from build123d import *

# Parameters (mm, degrees)
SKETCH1_R           = 2.5
BOSS_EXTRUDE1_DEPTH = 2


with BuildPart() as part:
    # Sketch1 → Boss-Extrude1 (new body)
    with BuildSketch(Plane(origin=(0, 0, 0), x_dir=(1, 0, 0), z_dir=(0, 1, 0))):
        with BuildLine():
            Line((0, 6), (110, 6))
            ThreePointArc((110, 6), (116, 0), (110, -6))
            Line((110, -6), (0, -6))
            ThreePointArc((0, -6), (-6, 0), (0, 6))
        make_face()
        with Locations(Location((0, 0, 0), (0, 0, 270))):
            Circle(SKETCH1_R, mode=Mode.SUBTRACT)
        with BuildLine():
            Line((10, 2), (110, 2))
            ThreePointArc((110, 2), (112, 0), (110, -2))
            Line((110, -2), (10, -2))
            ThreePointArc((10, -2), (8, 0), (10, 2))
        make_face(mode=Mode.SUBTRACT)
    extrude(amount=BOSS_EXTRUDE1_DEPTH)


solid = part.part
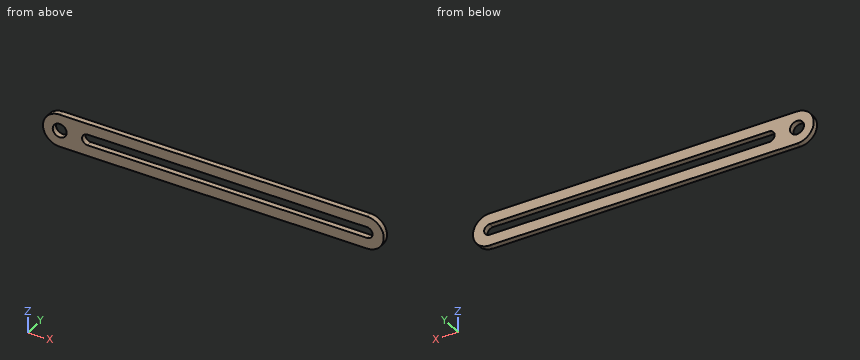
Input: part model. Units: mm. Frame: model coordinates. Coordinates: 2 decimals unless noted, no trailing zeros. Write each loop counter-clockwise with the first axis right and the second up, starting at its lowest first coordinate (ties: lowest second). Pieces come first, ordered by that corner, then holes. Notation, with made-up numbers: M 16.5,-0.75 L 38.5,-0.75 A27 cw 38.5,24.25 Z; hole C 39,-38.5 d2. An arc over 180 degrees is marked long. Answer as a JSON object with one key per item and string values. Group by question number.
(1) Section D-D on z = 4.5. Output: boundary loops of the cut face in (x, y), plus the area to 3 significant figures.
(2) Contact query for a flat-ended pin moving along its axis: P1, Ø1.5, axis at x = 19, z = 2, coming from the -Y side. Output: stop coordinate, or through.
(3) Section B-B on x = 77. Output: boundary loops of the cut face in (y, z), plus the area to 3 significant figures.
(4) Ray query, line 1 along X through (y, z) = (1, 0); line 2 along Z through (x, y) = (74.5, 1.45); line 3 along X through (y, z) = (0.35, -0.5). Return the intervals inside material, ascending. Write a range as [from, to].
(5) Section A-A on z = 0. Output: boundary loops of the cut face in (x, y), plus the area to 3 significant figures.
(6) Section C-C on y = 0.9. Output: boundary loops of the cut face in (x, z), plus the area to 3 significant figures.
Result set:
{
 "1": {"outline": "M -3.97,0 L 113.97,0 L 113.97,2 L -3.97,2 Z", "area": "236 mm2"},
 "2": {"P1": "stops at y = 0"},
 "3": {"outline": "M 0,-6 L 2,-6 L 2,-2 L 0,-2 Z; M 0,2 L 2,2 L 2,6 L 0,6 Z", "area": "16.0 mm2"},
 "4": {"line 1": "x = [-6, -2.5], [2.5, 8], [112, 116]", "line 2": "z = [-6, -2], [2, 6]", "line 3": "x = [-5.98, -2.45], [2.45, 8.06], [111.94, 115.98]"},
 "5": {"outline": "M -6,0 L -2.5,0 L -2.5,2 L -6,2 Z; M 2.5,0 L 8,0 L 8,2 L 2.5,2 Z; M 112,0 L 116,0 L 116,2 L 112,2 Z", "area": "26.0 mm2"},
 "6": {"outline": "M 0,-6 L 110,-6 A6 ccw 110,6 L 0,6 A6 ccw Z; hole C 0,0 d5; hole M 10,-2 L 110,-2 A2 ccw 110,2 L 10,2 A2 ccw Z", "area": "1,000 mm2"}
}
